CAD build for the part. Positions are in the model's coordinates, mm. Coordinates: 2 decimals unless noted, no trailing zeros. Loops run counter-clockwise (first coordinate to the right, second up) from the corner with the lowest first, then second, coordinate; pieces in that order, holes last.
1) Pin check, flat tips, straight feed: pin 1 Ø1 at (x, y) = (-4.5, 4) entering from -Z; pin 2 Ø8 at (y, z) = (-4, 3.5) entering from -X; pin 3 Ø2 at (x, z) = (3, -5.5) entering from +Y; pin 4 Ø3 at (y, z) = (-1.5, 6.5) entering from -X. Stop position of each tip, or through.
2) Saw through at C-C, the plane y = 0.5. Write the cut outline in (x, z).
3) Saw through at A-A, the plane z = 0. Write the cut outline in (x, y), and give its area (3 significant figures).
4) Wall check: line 1 along Z through (x, y) = (0, 2); line 2 along X through (y, z) = (6, -2); line 3 along Z through (x, y) = (0.75, -3.25). Give the ranges that are in metal, low to high.
5) Two-plate mould, pull along X, no slides. Class faces 1 (the cylindrical face through (-0.624, 4.008, 4.752)), 2 (the conical face through (4.803, 8.4, 1.513)): +X half, -X half, draft (parallel to the pull), parting line (faces both ways), or undercut.
6) Saw through at B-B, the plane x = 0. Write the cut outline in (y, z), and give its area (3 significant figures).
7) Saw through at D-D, the plane y = -1.25. Write the cut outline in (x, z).
```python
from build123d import *

# Parameters (mm, degrees)
F2_T = -5


# Not quite as in the source:
# - a fillet or chamfer that OpenCascade refuses, or shapes differently, is made with other operations: its cross-section is extruded or revolved along the edge and cut away or added


with BuildPart() as f1:
    # F0 (on Top) → F1 (revolve)
    with BuildSketch(Plane.XY):
        Polygon((0, 11.3076803427), (0, -11.3076803427), (9.7927384347, -5.6538401714), (9.7927384347, 5.6538401714), align=None)
    revolve(axis=Axis((0, 0, 0), (0, -1, 0)))

    # F2
    f2_openings = [f1.faces().sort_by_distance(p)[0] for p in [
        (-4.896369, -8.48076, 0),
        (-4.896369, 8.48076, 0),
    ]]
    offset(amount=F2_T, openings=f2_openings)

    # F3: fillet of radius 5 on 1 edges, made by hand

    # F3_s1 → F3_t2 (revolve, cut)
    with BuildSketch(Plane.XY):
        with BuildLine():
            ThreePointArc((9.7927384347, -5.6538401714), (6.2572045287, -4.1893740773), (4.7927384347, -0.6538401714))
            Line((4.7927384347, -0.6538401714), (4.6927384347, -0.6538401714))
            Line((4.6927384347, -0.6538401714), (4.6927384347, -8.5405915173))
            Line((4.6927384347, -8.5405915173), (4.8427384347, -8.6271940577))
            ThreePointArc((4.8427384347, -8.6271940577), (7.3427384347, -7.1838183847), (9.7927384347, -5.7538401714))
            Line((9.7927384347, -5.7538401714), (9.7927384347, -5.6538401714))
        make_face()
    revolve(axis=Axis((0, -8.5405915173, 0), (0, 1, 0)), mode=Mode.SUBTRACT)


solid = f1.part
```
Data:
1. pin 1: stops at z = -8.94
1. pin 2: stops at x = -9.79
1. pin 3: stops at y = 8.27
1. pin 4: stops at x = -8.42
2. outline: circle Ø19.59 at (0, 0); hole circle Ø9.59 at (0, 0)
3. outline: (-9.79, -5.65) arc R5 ccw to (-4.79, -0.65) - (-4.79, 8.54) - (-9.79, 5.65) - close; (4.79, -0.65) arc R5 ccw to (9.79, -5.65) - (9.79, 5.65) - (4.79, 8.54) - close
3. area: 117 mm2
4. line 1: z = -9.79 to -4.79, 4.79 to 9.79
4. line 2: x = -8.97 to -4.36, 4.36 to 8.97
4. line 3: z = -9.76 to -5.47, 5.47 to 9.76
5. face 1: undercut
5. face 2: parting line
6. outline: (-5.65, -9.79) - (5.65, -9.79) - (8.54, -4.79) - (-0.65, -4.79) arc R5 ccw to start; (-5.65, 9.79) arc R5 ccw to (-0.65, 4.79) - (8.54, 4.79) - (5.65, 9.79) - close
6. area: 117 mm2
7. outline: circle Ø19.59 at (0, 0); hole circle Ø9.66 at (0, 0)
